```python
from build123d import *

# Parameters (mm, degrees)
EXTRUDE_1_DEPTH     = 119.5
CUT_EXTRUDE_1_DEPTH = 115.5
SKETCH_3_R          = 1.4
CUT_EXTRUDE_2_DEPTH = 4
EXTRUDE_2_DEPTH     = 2.5
EXTRUDE_3_DEPTH     = 2.5
CUT_EXTRUDE_3_DEPTH = 31.4
CHAMFER_1_SIZE      = 0.4
SKETCH_3_3_R        = 1.4
CUT_EXTRUDE_4_DEPTH = 2.5
SKETCH_3_4_R        = 1.4
CUT_EXTRUDE_5_DEPTH = 4
SKETCH_9_R          = 1.6
CUT_EXTRUDE_6_DEPTH = 148.893469266
CHAMFER_4_SIZE      = 0.4
CHAMFER_5_SIZE      = 0.4


with BuildPart() as part:
    # Sketch 1 → Extrude 1 (new body)
    with BuildSketch(Plane.XY):
        with BuildLine():
            Line((-38.75609893, 20.654436608), (39.89390107, 20.654436608))
            ThreePointArc((39.89390107, 20.654436608), (42.015221413, 19.775756952), (42.89390107, 17.654436608))
            Line((42.89390107, 17.654436608), (42.89390107, -16.745563392))
            ThreePointArc((42.89390107, -16.745563392), (42.015221413, -18.866883735), (39.89390107, -19.745563392))
            Line((39.89390107, -19.745563392), (-38.75609893, -19.745563392))
            ThreePointArc((-38.75609893, -19.745563392), (-40.877419274, -18.866883735), (-41.75609893, -16.745563392))
            Line((-41.75609893, -16.745563392), (-41.75609893, 17.654436608))
            ThreePointArc((-41.75609893, 17.654436608), (-40.877419274, 19.775756952), (-38.75609893, 20.654436608))
        make_face()
    extrude(amount=EXTRUDE_1_DEPTH)

    # Sketch 2 → Cut-Extrude 1 (cut)
    with BuildSketch(Plane.XY.offset(119.5)):
        with BuildLine():
            Line((-37.75609893, 16.654436608), (38.89390107, 16.654436608))
            Line((38.89390107, 16.654436608), (38.89390107, -14.745563392))
            Line((38.89390107, -14.745563392), (37.319829514, -14.745563392))
            ThreePointArc((37.319829514, -14.745563392), (37.022296896, -14.866580802), (36.893704546, -15.160918839))
            ThreePointArc((36.893704546, -15.160918839), (36.712700981, -15.575222133), (36.29390107, -15.745563392))
            Line((36.29390107, -15.745563392), (-35.15609893, -15.745563392))
            ThreePointArc((-35.15609893, -15.745563392), (-35.580362999, -15.56982746), (-35.75609893, -15.145563392))
            Line((-35.75609893, -15.145563392), (-35.75609893, -15.142198174))
            ThreePointArc((-35.75609893, -15.142198174), (-35.868562438, -14.862087147), (-36.147008919, -14.745563392))
            Line((-36.147008919, -14.745563392), (-37.75609893, -14.745563392))
            Line((-37.75609893, -14.745563392), (-37.75609893, 16.654436608))
        make_face()
    extrude(amount=-CUT_EXTRUDE_1_DEPTH, mode=Mode.SUBTRACT)

    # Sketch 3 → Cut-Extrude 2 (cut)
    with BuildSketch(Plane.XY.offset(4)):
        with BuildLine():
            Line((29.39390107, 16.654436608), (-28.25609893, 16.654436608))
            Line((-28.25609893, 16.654436608), (-28.25609893, 12.454436608))
            ThreePointArc((-28.25609893, 12.454436608), (-29.281225196, 9.979562874), (-31.75609893, 8.954436608))
            Line((-31.75609893, 8.954436608), (-37.75609893, 8.954436608))
            Line((-37.75609893, 8.954436608), (-37.75609893, -7.045563392))
            Line((-37.75609893, -7.045563392), (-31.75609893, -7.045563392))
            ThreePointArc((-31.75609893, -7.045563392), (-29.281225196, -8.070689657), (-28.25609893, -10.545563392))
            Line((-28.25609893, -10.545563392), (-28.25609893, -15.745563392))
            Line((-28.25609893, -15.745563392), (29.39390107, -15.745563392))
            Line((29.39390107, -15.745563392), (29.39390107, -10.545563392))
            ThreePointArc((29.39390107, -10.545563392), (30.419027336, -8.070689657), (32.89390107, -7.045563392))
            Line((32.89390107, -7.045563392), (38.89390107, -7.045563392))
            Line((38.89390107, -7.045563392), (38.89390107, 8.954436608))
            Line((38.89390107, 8.954436608), (32.89390107, 8.954436608))
            ThreePointArc((32.89390107, 8.954436608), (30.419027336, 9.979562874), (29.39390107, 12.454436608))
            Line((29.39390107, 12.454436608), (29.39390107, 16.654436608))
        make_face()
        with Locations((-31.75609893, -10.545563392)):
            Circle(SKETCH_3_R)
        with Locations((32.89390107, 12.454436608)):
            Circle(SKETCH_3_R)
        with Locations((32.89390107, -10.545563392)):
            Circle(SKETCH_3_R)
    extrude(amount=-CUT_EXTRUDE_2_DEPTH, mode=Mode.SUBTRACT)

    # Sketch 4 → Extrude 2 (add)
    with BuildSketch(Plane.ZY.offset(-38.89390107)):
        Polygon((19.4, 3.254436608), (97.4, 3.254436608), (99.4, 1.254436608), (99.4, 0.654436608), (97.4, -1.345563392), (19.4, -1.345563392), align=None)
        Polygon((20.146290163, 16.654436608), (99.4, 16.654436608), (99.4, 15.654436608), (97.4, 13.654436608), (20.146290163, 13.654436608), align=None)
        Polygon((19.4, -11.745563392), (97.4, -11.745563392), (99.4, -13.745563392), (99.4, -15.145563392), (19.4, -15.145563392), align=None)
    extrude(amount=EXTRUDE_2_DEPTH)

    # Sketch 6 → Extrude 3 (add)
    with BuildSketch(Plane(origin=(-37.75609893, 0, 0), x_dir=(0, 0, -1), z_dir=(1, 0, 0))):
        Polygon((-99.4, 16.654436608), (-19.4, 16.654436608), (-19.4, 13.654436608), (-97.4, 13.654436608), (-99.4, 15.654436608), align=None)
        Polygon((-97.4, 3.254436608), (-19.4, 3.254436608), (-19.4, -1.345563392), (-97.4, -1.345563392), (-99.4, 0.654436608), (-99.4, 1.254436608), align=None)
        Polygon((-97.4, -11.745563392), (-19.4, -11.745563392), (-19.4, -15.145563392), (-99.4, -15.145563392), (-99.4, -13.745563392), align=None)
    extrude(amount=EXTRUDE_3_DEPTH)

    # Sketch 8 → Cut-Extrude 3 (cut)
    with BuildSketch(Plane.XZ.offset(-16.654436608)):
        with BuildLine():
            Line((-39.75609893, 114.19), (-39.75609893, 119.5))
            Line((-39.75609893, 119.5), (-34.75609893, 119.5))
            Line((-34.75609893, 119.5), (-34.75609893, 107.305312266))
            Line((-34.75609893, 107.305312266), (-37.75609893, 107.305312266))
            ThreePointArc((-37.75609893, 107.305312266), (-37.902054498, 108.229666299), (-38.325719183, 109.064077255))
            ThreePointArc((-38.325719183, 109.064077255), (-38.505927368, 109.602965716), (-38.346327705, 110.148313046))
            ThreePointArc((-38.346327705, 110.148313046), (-38.025073016, 111.013058128), (-38.12609893, 111.93))
            ThreePointArc((-38.12609893, 111.93), (-38.780481743, 113.175843369), (-39.75609893, 114.19))
        make_face()
        with BuildLine():
            Line((38.89390107, 107.18052563), (35.89390107, 107.18052563))
            Line((35.89390107, 107.18052563), (35.89390107, 119.5))
            Line((35.89390107, 119.5), (40.89390107, 119.5))
            Line((40.89390107, 119.5), (40.89390107, 114.19))
            ThreePointArc((40.89390107, 114.19), (39.886150452, 113.181702896), (39.20390107, 111.93))
            ThreePointArc((39.20390107, 111.93), (39.097168141, 110.960326838), (39.461822803, 110.055514737))
            ThreePointArc((39.461822803, 110.055514737), (39.64389997, 109.497678446), (39.463521323, 108.939290618))
            ThreePointArc((39.463521323, 108.939290618), (39.039856638, 108.104879663), (38.89390107, 107.18052563))
        make_face()
    extrude(amount=CUT_EXTRUDE_3_DEPTH, mode=Mode.SUBTRACT)

    # Chamfer 1
    chamfer_1_edges = [part.edges().sort_by_distance(p)[0] for p in [
        (0.56890107, -19.745563392, 0),
        (-40.877419274, -18.866883735, 0),
        (-41.75609893, 0.454436608, 0),
        (-40.877419274, 19.775756952, 0),
        (0.56890107, 20.654436608, 0),
        (42.015221413, 19.775756952, 0),
        (42.89390107, 0.454436608, 0),
        (42.015221413, -18.866883735, 0),
    ]]
    chamfer(chamfer_1_edges, length=CHAMFER_1_SIZE)

    # Sketch 3_3 → Cut-Extrude 4 (cut)
    with BuildSketch(Plane.XY.offset(4)):
        with Locations((-31.75609893, -10.545563392)):
            Circle(SKETCH_3_3_R)
        with Locations((32.89390107, 12.454436608)):
            Circle(SKETCH_3_3_R)
        with Locations((32.89390107, -10.545563392)):
            Circle(SKETCH_3_3_R)
        with Locations((-31.75609893, 12.454436608)):
            Circle(SKETCH_3_3_R)
        with BuildLine():
            Line((-28.25609893, 16.654436608), (29.39390107, 16.654436608))
            Line((29.39390107, 16.654436608), (29.39390107, 12.454436608))
            ThreePointArc((29.39390107, 12.454436608), (30.419027336, 9.979562874), (32.89390107, 8.954436608))
            Line((32.89390107, 8.954436608), (38.89390107, 8.954436608))
            Line((38.89390107, 8.954436608), (38.89390107, -7.045563392))
            Line((38.89390107, -7.045563392), (32.89390107, -7.045563392))
            ThreePointArc((32.89390107, -7.045563392), (30.419027336, -8.070689657), (29.39390107, -10.545563392))
            Line((29.39390107, -10.545563392), (29.39390107, -15.745563392))
            Line((29.39390107, -15.745563392), (-28.25609893, -15.745563392))
            Line((-28.25609893, -15.745563392), (-28.25609893, -10.545563392))
            ThreePointArc((-28.25609893, -10.545563392), (-29.281225196, -8.070689657), (-31.75609893, -7.045563392))
            Line((-31.75609893, -7.045563392), (-37.75609893, -7.045563392))
            Line((-37.75609893, -7.045563392), (-37.75609893, 8.954436608))
            Line((-37.75609893, 8.954436608), (-31.75609893, 8.954436608))
            ThreePointArc((-31.75609893, 8.954436608), (-29.281225196, 9.979562874), (-28.25609893, 12.454436608))
            Line((-28.25609893, 12.454436608), (-28.25609893, 16.654436608))
        make_face()
    extrude(amount=-CUT_EXTRUDE_4_DEPTH, mode=Mode.SUBTRACT)

    # Sketch 3_4 → Cut-Extrude 5 (cut)
    with BuildSketch(Plane.XY.offset(4)):
        with Locations((-31.75609893, -10.545563392)):
            Circle(SKETCH_3_4_R)
        with Locations((32.89390107, 12.454436608)):
            Circle(SKETCH_3_4_R)
        with Locations((32.89390107, -10.545563392)):
            Circle(SKETCH_3_4_R)
        with Locations((-31.75609893, 12.454436608)):
            Circle(SKETCH_3_4_R)
        with BuildLine():
            Line((-28.25609893, 16.654436608), (29.39390107, 16.654436608))
            Line((29.39390107, 16.654436608), (29.39390107, 12.454436608))
            ThreePointArc((29.39390107, 12.454436608), (30.419027336, 9.979562874), (32.89390107, 8.954436608))
            Line((32.89390107, 8.954436608), (38.89390107, 8.954436608))
            Line((38.89390107, 8.954436608), (38.89390107, -7.045563392))
            Line((38.89390107, -7.045563392), (32.89390107, -7.045563392))
            ThreePointArc((32.89390107, -7.045563392), (30.419027336, -8.070689657), (29.39390107, -10.545563392))
            Line((29.39390107, -10.545563392), (29.39390107, -15.745563392))
            Line((29.39390107, -15.745563392), (-28.25609893, -15.745563392))
            Line((-28.25609893, -15.745563392), (-28.25609893, -10.545563392))
            ThreePointArc((-28.25609893, -10.545563392), (-29.281225196, -8.070689657), (-31.75609893, -7.045563392))
            Line((-31.75609893, -7.045563392), (-37.75609893, -7.045563392))
            Line((-37.75609893, -7.045563392), (-37.75609893, 8.954436608))
            Line((-37.75609893, 8.954436608), (-31.75609893, 8.954436608))
            ThreePointArc((-31.75609893, 8.954436608), (-29.281225196, 9.979562874), (-28.25609893, 12.454436608))
            Line((-28.25609893, 12.454436608), (-28.25609893, 16.654436608))
        make_face()
    extrude(amount=-CUT_EXTRUDE_5_DEPTH, mode=Mode.SUBTRACT)

    # Sketch 9 → Cut-Extrude 6 (cut, through all)
    with BuildSketch(Plane(origin=(42.89390107, 0, 0), x_dir=(0, 0, -1), z_dir=(1, 0, 0))):
        with Locations(Location((-89.5, 0.954436608, 0), (0, 0, 90))):
            Circle(SKETCH_9_R)
        with Locations(Location((-30, 0.954436608, 0), (0, 0, 90))):
            Circle(SKETCH_9_R)
    extrude(amount=-CUT_EXTRUDE_6_DEPTH, mode=Mode.SUBTRACT)

    # Chamfer 4
    chamfer_4_edges = [part.edges().sort_by_distance(p)[0] for p in [
        (-33.15609893, 12.454436608, 0),
        (-33.15609893, -10.545563392, 0),
        (31.49390107, 12.454436608, 0),
        (31.49390107, -10.545563392, 0),
        (35.89390107, 8.954436608, 0),
        (38.89390107, 0.954436608, 0),
        (35.89390107, -7.045563392, 0),
        (0.56890107, -15.745563392, 0),
        (-28.25609893, -13.145563392, 0),
        (-34.75609893, -7.045563392, 0),
        (-37.75609893, 0.954436608, 0),
        (-34.75609893, 8.954436608, 0),
        (0.56890107, 16.654436608, 0),
        (29.39390107, 14.554436608, 0),
        (30.419027336, 9.979562874, 0),
        (30.419027336, -8.070689657, 0),
        (29.39390107, -13.145563392, 0),
        (-29.281225196, -8.070689657, 0),
        (-29.281225196, 9.979562874, 0),
        (-28.25609893, 14.554436608, 0),
    ]]
    chamfer(chamfer_4_edges, length=CHAMFER_4_SIZE)

    # Chamfer 5
    chamfer_5_edges = [part.edges().sort_by_distance(p)[0] for p in [
        (-33.15609893, 12.454436608, 4),
        (-33.15609893, -10.545563392, 4),
        (31.49390107, 12.454436608, 4),
        (31.49390107, -10.545563392, 4),
        (30.419027336, 9.979562874, 4),
        (30.419027336, -8.070689657, 4),
        (29.39390107, -13.145563392, 4),
        (-29.281225196, -8.070689657, 4),
        (-29.281225196, 9.979562874, 4),
        (-28.25609893, 14.554436608, 4),
        (29.39390107, 14.554436608, 4),
        (-34.75609893, 8.954436608, 4),
        (-34.75609893, -7.045563392, 4),
        (-28.25609893, -13.145563392, 4),
        (35.89390107, -7.045563392, 4),
        (35.89390107, 8.954436608, 4),
    ]]
    chamfer(chamfer_5_edges, length=CHAMFER_5_SIZE)


solid = part.part
```
Could you check a few things on this model? Use its own coordinates, in mm. A direction names the side the tool comes from. Give positions to 0.01 mm unless a question says otherwise; leave off trailing zeros. Loops run counter-clockwise (first coordinate to the right, second up) from the corner with the lowest first, then second, coordinate; pieces in that order, holes last. Notation, with made-up numbers: (-21.5, 59.25) - (-16.5, 59.25) arc R37 ccw to (-16.5, 97.25) - close; hole circle Ø10 at (69.25, -5.75). An arc over 180 degrees is marked (long way). Answer in a Markdown table with one row per item. Add a question column.
Q1. For pin 1 (6.5 mm diameter, centred on x = 35, y = -10.5, fed in from +Z); pin 2 (6 mm diameter, centred on x = 35.5, y = 12, fed in from +Z); pin 3 (4 mm diameter, centred on x = -35, y = -12, fed in from +Z), each with a flat end and sliding along its axis, tell me the tip position at first contact or that it passes through.
Q2. If we section it at A-A (x = 25): List the corners of the cut face in (y, z) for me.
Q3. Please list where these lines run through material, in increasing order: L1, parallel to Y at x = -37, z = 89.5; L2, parallel to Y at x = 38, z = 45; L3, parallel to Y at x = -4.5, z = 105. Write a range as from..to.
Q4. Which directions (+Z, -Z, +X, -X, +Y, -Y) give clear straight access to the entire face, cutting with the end or side of a thin tool? Please do faces 1 (the face through (30.6, -8.3, 3.89)), 2 (the face through (-29.46, 10.21, 0.11)), 3 (the face through (-40.654, -18.686, 0.114)), 4 (the face through (-40.696, 19.552, 0.114)), 5 (the face through (30.39, -8.1, 2.02)).
Q5. We'd pull the mould along Z, two halves only. Please class faces 6 (the face through (36.394, 1, 60)), 7 (the face through (-38.461, 0.746, 31.586)), 8 (the face through (-29.51, -8.25, 0.11)): +Z half, -Z half, draft (parallel to the pull), parting line (faces both ways), or undercut.
The answers:
| question | item | result |
|---|---|---|
| 1 | pin 1 | stops at z = 99.09 |
| 1 | pin 2 | stops at z = 98.61 |
| 1 | pin 3 | stops at z = 99.4 |
| 2 | outline | (-19.75, 0.4) - (-19.35, 0) - (-16.15, 0) - (-15.75, 0.4) - (-15.75, 119.5) - (-19.75, 119.5) - close; (16.65, 0.4) - (17.05, 0) - (20.25, 0) - (20.65, 0.4) - (20.65, 119.5) - (16.65, 119.5) - close |
| 3 | L1 | y = -19.75..-11.75, -1.35..-0.65, 2.55..3.25, 13.65..20.65 |
| 3 | L2 | y = -19.75..-11.75, -1.35..3.25, 13.65..20.65 |
| 3 | L3 | y = -19.75..-15.75, 16.65..20.65 |
| 4 | face 1 | +Z |
| 4 | face 2 | -Z |
| 4 | face 3 | -Z, -X, -Y |
| 4 | face 4 | -Z, -X, +Y |
| 4 | face 5 | +Z, -Z |
| 5 | face 6 | draft |
| 5 | face 7 | undercut |
| 5 | face 8 | -Z half |
